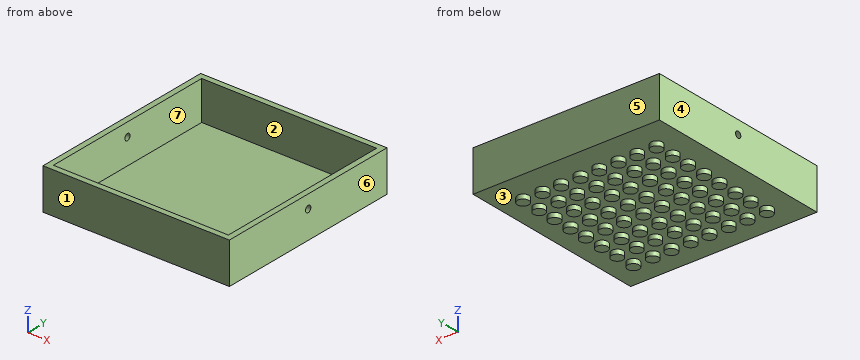
```python
from build123d import *

# Parameters (mm, degrees)
F0_W     = 77.190011016
F0_H     = 79.099989416
F0_W_2   = 72.470011016
F0_H_2   = 74.379989416
F1_DEPTH = 16.95
F2_W     = 79.099989416
F2_H     = 0.9
F3_DEPTH = 74.830011016
F4_R     = 1.33
F5_DEPTH = 77.191011016
F6_R     = 2.3749
F7_DEPTH = 1.8288


with BuildPart() as f1:
    # F0 (on Top) → F1 (new body)
    with BuildSketch(Plane.XY):
        Rectangle(F0_W, F0_H)
        Rectangle(F0_W_2, F0_H_2, mode=Mode.SUBTRACT)
    extrude(amount=F1_DEPTH)

    # F2 (on face) → F3 (join, through all)
    with BuildSketch(Plane(origin=(-38.595005508, 0, 0), x_dir=(0, -1, 0), z_dir=(-1, 0, 0))):
        with Locations((0, 0.45)):
            Rectangle(F2_W, F2_H)
    extrude(amount=-F3_DEPTH)

    # F4 (on face) → F5 (cut, through all)
    with BuildSketch(Plane(origin=(-38.595005508, 0, 0), x_dir=(0, -1, 0), z_dir=(-1, 0, 0))):
        with Locations((0, 11.424992)):
            Circle(F4_R)
    extrude(amount=-F5_DEPTH, mode=Mode.SUBTRACT)

    # F6 (on face) → F7 (join)
    with BuildSketch(Plane(origin=(0, 0, 0), x_dir=(1, 0, 0), z_dir=(0, 0, -1))):
        with Locations((-27.6479, 27.6479)):
            Circle(F6_R)
        with Locations((-19.5961, 27.6479)):
            Circle(F6_R)
        with Locations((-11.8999, 27.6479)):
            Circle(F6_R)
        with Locations((-3.8481, 27.6479)):
            Circle(F6_R)
        with Locations((3.8481, 27.6479)):
            Circle(F6_R)
        with Locations((11.8999, 27.6479)):
            Circle(F6_R)
        with Locations((19.5961, 27.6479)):
            Circle(F6_R)
        with Locations((27.6479, 27.6479)):
            Circle(F6_R)
        with Locations((27.6479, 19.5961)):
            Circle(F6_R)
        with Locations((19.5961, 19.5961)):
            Circle(F6_R)
        with Locations((11.8999, 19.5961)):
            Circle(F6_R)
        with Locations((3.8481, 19.5961)):
            Circle(F6_R)
        with Locations((-3.8481, 19.5961)):
            Circle(F6_R)
        with Locations((-11.8999, 19.5961)):
            Circle(F6_R)
        with Locations((-19.5961, 19.5961)):
            Circle(F6_R)
        with Locations((-27.6479, 19.5961)):
            Circle(F6_R)
        with Locations((-27.6479, 11.8999)):
            Circle(F6_R)
        with Locations((-19.5961, 11.8999)):
            Circle(F6_R)
        with Locations((-11.8999, 11.8999)):
            Circle(F6_R)
        with Locations((-3.8481, 11.8999)):
            Circle(F6_R)
        with Locations((3.8481, 11.8999)):
            Circle(F6_R)
        with Locations((11.8999, 11.8999)):
            Circle(F6_R)
        with Locations((19.5961, 11.8999)):
            Circle(F6_R)
        with Locations((27.6479, 11.8999)):
            Circle(F6_R)
        with Locations((27.6479, 3.8481)):
            Circle(F6_R)
        with Locations((19.5961, 3.8481)):
            Circle(F6_R)
        with Locations((11.8999, 3.8481)):
            Circle(F6_R)
        with Locations((3.8481, 3.8481)):
            Circle(F6_R)
        with Locations((-3.8481, 3.8481)):
            Circle(F6_R)
        with Locations((-11.8999, 3.8481)):
            Circle(F6_R)
        with Locations((-19.5961, 3.8481)):
            Circle(F6_R)
        with Locations((-27.6479, 3.8481)):
            Circle(F6_R)
        with Locations((-27.6479, -3.8481)):
            Circle(F6_R)
        with Locations((-19.5961, -3.8481)):
            Circle(F6_R)
        with Locations((-11.8999, -3.8481)):
            Circle(F6_R)
        with Locations((-3.8481, -3.8481)):
            Circle(F6_R)
        with Locations((3.8481, -3.8481)):
            Circle(F6_R)
        with Locations((11.8999, -3.8481)):
            Circle(F6_R)
        with Locations((19.5961, -3.8481)):
            Circle(F6_R)
        with Locations((27.6479, -3.8481)):
            Circle(F6_R)
        with Locations((27.6479, -11.8999)):
            Circle(F6_R)
        with Locations((19.5961, -11.8999)):
            Circle(F6_R)
        with Locations((11.8999, -11.8999)):
            Circle(F6_R)
        with Locations((3.8481, -11.8999)):
            Circle(F6_R)
        with Locations((-3.8481, -11.8999)):
            Circle(F6_R)
        with Locations((-11.8999, -11.8999)):
            Circle(F6_R)
        with Locations((-19.5961, -11.8999)):
            Circle(F6_R)
        with Locations((-27.6479, -11.8999)):
            Circle(F6_R)
        with Locations((-27.6479, -19.5961)):
            Circle(F6_R)
        with Locations((-19.5961, -19.5961)):
            Circle(F6_R)
        with Locations((-11.8999, -19.5961)):
            Circle(F6_R)
        with Locations((-3.8481, -19.5961)):
            Circle(F6_R)
        with Locations((3.8481, -19.5961)):
            Circle(F6_R)
        with Locations((11.8999, -19.5961)):
            Circle(F6_R)
        with Locations((19.5961, -19.5961)):
            Circle(F6_R)
        with Locations((27.6479, -19.5961)):
            Circle(F6_R)
        with Locations((27.6479, -27.6479)):
            Circle(F6_R)
        with Locations((19.5961, -27.6479)):
            Circle(F6_R)
        with Locations((11.8999, -27.6479)):
            Circle(F6_R)
        with Locations((3.8481, -27.6479)):
            Circle(F6_R)
        with Locations((-3.8481, -27.6479)):
            Circle(F6_R)
        with Locations((-11.8999, -27.6479)):
            Circle(F6_R)
        with Locations((-19.5961, -27.6479)):
            Circle(F6_R)
        with Locations((-27.6479, -27.6479)):
            Circle(F6_R)
    extrude(amount=F7_DEPTH)


solid = f1.part
```
Geometry: final body of the model. Coordinates: model frame, mm. Face numbers are marked on the shaded views. A direction names the side the tool comes from. Give positions to 0.01 mm unless a question says otherwise; leave off trailing zeros. Loops run counter-clockwise (first coordinate to the right, second up) from the corner with the lowest first, then second, coordinate; pieces in that order, holes last. Notation, with made-up numbers: (27, 86) -> (48, 86) arc R24 ccw to (48, 109) -> close; hole circle Ø2 at (-24, 11). An arc over 180 degrees is marked (long way). Return JSON: item names as keys, results as strings.
Item 1: Section B-B, the plane y = 0. Output: boundary loops of the cut face in (x, z) (3 decimals), plus the area to 3 significant figures.
Filled in:
{"outline": "(-38.595, 0) -> (38.595, 0) -> (38.595, 10.095) -> (36.235, 10.095) -> (36.235, 0.9) -> (-36.235, 0.9) -> (-36.235, 10.095) -> (-38.595, 10.095) -> close; (-38.595, 12.755) -> (-36.235, 12.755) -> (-36.235, 16.95) -> (-38.595, 16.95) -> close; (36.235, 12.755) -> (38.595, 12.755) -> (38.595, 16.95) -> (36.235, 16.95) -> close", "area": "133 mm^2"}
Item 2: Section A-A, the plane z = 8.75. Output: boundary loops of the cut face in (x, y) (3 decimals), plus the area to 3 significant figures.
Filled in:
{"outline": "(-38.595, -39.55) -> (38.595, -39.55) -> (38.595, 39.55) -> (-38.595, 39.55) -> close; hole (-36.235, -37.19) -> (36.235, -37.19) -> (36.235, 37.19) -> (-36.235, 37.19) -> close", "area": "715 mm^2"}
Item 3: Section C-C, the plane x = -23. Output: boundary loops of the cut face in (y, z).
Filled in:
{"outline": "(-39.55, 0) -> (39.55, 0) -> (39.55, 16.95) -> (37.19, 16.95) -> (37.19, 0.9) -> (-37.19, 0.9) -> (-37.19, 16.95) -> (-39.55, 16.95) -> close"}
Item 4: Section D-D, the plane y = 31. Output: boundary loops of the cut face in (x, z) (3 decimals), plus the area to 3 significant figures.
Filled in:
{"outline": "(-38.595, 0) -> (38.595, 0) -> (38.595, 16.95) -> (36.235, 16.95) -> (36.235, 0.9) -> (-36.235, 0.9) -> (-36.235, 16.95) -> (-38.595, 16.95) -> close", "area": "145 mm^2"}
Item 5: Access query for the marked faces 1, 2 and 3. Directions: +Z, -Z, +X, -X, +Y, -Y. A direction counts if a zero-diameter tool reaches every point of the face in a straight line with its end or side. Return the directions, or none.
Filled in:
{"face 1": "+Z, -Z, +X, -X, -Y", "face 2": "+Z", "face 3": "-Z"}
Item 6: Pin query (flat end, axial travel): P1, Ø1, axis at x = 15.5, y = 21, coming from the -Z side; P2, Ø4, axis at x = -3, y = -3, coming from the +Z side; P3, Ø23, axis at x = 1, y = -1, coming from the -Z side. Return the tip coordinate at first contact, or that it passes through.
Filled in:
{"P1": "z = 0", "P2": "z = 0.9", "P3": "z = -1.83"}
Item 7: Line query: line 1 (X direction, y = 19, z = 8.25) (3 decimals); line 2 (Y direction, x = 16.5, z = 6); line 3 (Z direction, x = -37, y = 0) (3 decimals). Output: solid intervals per line, ascending.
Filled in:
{"line 1": "-38.595 to -36.235, 36.235 to 38.595", "line 2": "-39.55 to -37.19, 37.19 to 39.55", "line 3": "0 to 10.095, 12.755 to 16.95"}
Item 8: Mould query, pull axis X, two halves, no side actions, for the marked faces 4, 5, 6 and 7. Classes: released by +X, released by -X, zero draft, split by the parting line, or undercut.
Filled in:
{"face 4": "released by -X", "face 5": "zero draft", "face 6": "released by +X", "face 7": "undercut"}
